from build123d import *

# Parameters (mm, degrees)
EXTRUDE_1_DEPTH     = 5
EXTRUDE_2_DEPTH     = 6
EXTRUDE_3_DEPTH     = 6
SKETCH_4_R          = 8
CUT_EXTRUDE_1_DEPTH = 39.963875359


with BuildPart() as part:
    # 草图1 → 凸台-拉伸1 (new, symmetric)
    with BuildSketch(Plane.XY):
        with BuildLine():
            ThreePointArc((17.364205719, 2.386345678), (19.534538398, -5.841979928), (27.889014085, -7.460133888))
            ThreePointArc((27.889014085, -7.460133888), (32.219400839, -3.446774076), (32.617548437, 2.443963137))
            ThreePointArc((32.617548437, 2.443963137), (24.999999643, 9.4528e-05), (17.364205719, 2.386345678))
        make_face()
        with BuildLine():
            ThreePointArc((-0.737142857, 14.981876398), (-10.864095518, 10.342699288), (-15, 0))
            Line((-15, 0), (-15, -13.8873794))
            ThreePointArc((-15, -13.8873794), (-14.015653031, -16.10934764), (-11.708571429, -16.873190745))
            ThreePointArc((-11.708571429, -16.873190745), (8.410971794, -13.51595237), (27.889014085, -7.460133888))
            ThreePointArc((27.889014085, -7.460133888), (19.534538398, -5.841979928), (17.364205719, 2.386345678))
            ThreePointArc((17.364205719, 2.386345678), (13.547023493, 6.501980338), (11.776397664, 11.828725402))
            ThreePointArc((11.776397664, 11.828725402), (10.960769899, 13.5814964), (9.245219778, 14.472755399))
            ThreePointArc((9.245219778, 14.472755399), (4.266792486, 14.97738476), (-0.737142857, 14.981876398))
        make_face()
    extrude(amount=EXTRUDE_1_DEPTH, both=True)

    # 草图2 → 凸台-拉伸2 (add, symmetric)
    with BuildSketch(Plane.XY):
        with BuildLine():
            ThreePointArc((-15, 0), (3.625161022, -14.555349792), (13.247761009, 7.03539823))
            ThreePointArc((13.247761009, 7.03539823), (7.410500688, 13.041644051), (-0.737142857, 14.981876398))
            ThreePointArc((-0.737142857, 14.981876398), (-10.864095518, 10.342699288), (-15, 0))
        make_face()
    extrude(amount=EXTRUDE_2_DEPTH, both=True)

    # 草图3 → 凸台-拉伸3 (add, symmetric)
    with BuildSketch(Plane.XY):
        with BuildLine():
            ThreePointArc((17.364205719, 2.386345678), (25.030218713, -7.999942927), (32.617548437, 2.443963137))
            ThreePointArc((32.617548437, 2.443963137), (24.999999643, 9.4528e-05), (17.364205719, 2.386345678))
        make_face()
    extrude(amount=EXTRUDE_3_DEPTH, both=True)

    # 草图4 → 切除-拉伸1 (cut, through all)
    with BuildSketch(Plane.XY.offset(6)):
        Circle(SKETCH_4_R)
    extrude(amount=-CUT_EXTRUDE_1_DEPTH, mode=Mode.SUBTRACT)


solid = part.part
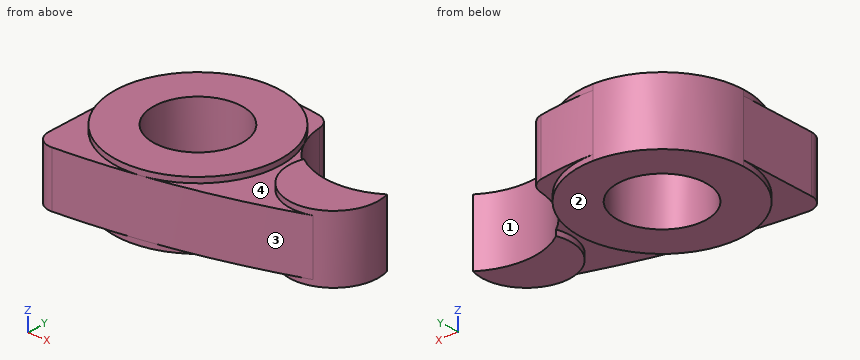
Geometry: final body of the model. Coordinates: model frame, mm. Face numbers are marked on the shaded views. Give positions to 0.01 mm unless a question says otherwise; leave off trailing zeros. Write each loop counter-clockwise with the first axis right and the second up, starting at its lowest first coordinate (ties: lowest second). Pieces come first, ordered by that corner, then holes. Notation, with made-up numbers: (41, 57.5) -> (84, 57.5) arc R14 ccw to (84, 69.5) -> close; hole circle Ø2 at (87, -24). An arc over 180 degrees is marked (long way). Answer as a JSON object with one key per item and string values.
1. Ray query, probe 1 along Z at (x, y) = (15.5, -3.5); probe 2 along Y at (x, z) = (0, -0.25); probe 3 along Y at (x, z) = (-7, 4). Return the intervals inside material, ascending. Write a range as from..to.
Ans:
{"probe 1": "z = -5..5", "probe 2": "y = -15.26..-8, 8..15.01", "probe 3": "y = -16.34..-3.87, 3.87..13.27"}
2. Contact query for flat-ended pins moving along their axis: pin 1 (2 mm diameter, centred on y = 5.5, z = -2.5, fed in from +X); pin 2 (4 mm diameter, centred on x = 16.5, z = 4, fed in from +Y). Output: stop coordinate, or through.
Ans:
{"pin 1": "stops at x = 15", "pin 2": "stops at y = 5.1"}
3. Cut plane A-A on z = -0.5. Output: boundary loops of the cut face in (x, y), and give its area (3 significant figures).
Ans:
{"outline": "(-15, -13.89) arc R3 ccw to (-11.71, -16.87) arc R150 ccw to (27.89, -7.46) arc R8 ccw to (32.62, 2.44) arc R13.25 cw to (11.78, 11.83) arc R3 ccw to (9.25, 14.47) arc R50 ccw to (-0.74, 14.98) arc R15 ccw to (-15, 0) -> close; hole circle Ø16 at (0, 0)", "area": "792 mm^2"}
4. Mould query, pull axis X, two halves, no side actions, for the marked faces 1, 2, 3 and 4. Classes: pulls with the +X half, pulls with the -X half, needs draft (parallel to the pull), parting line crosses it, or undercut.
Ans:
{"face 1": "undercut", "face 2": "needs draft", "face 3": "pulls with the +X half", "face 4": "undercut"}
5. Cut plane B-B on x = 5. Output: boundary loops of the cut face in (y, z) (3 decimals).
Ans:
{"outline": "(-14.285, -5) -> (-14.142, -5) -> (-14.142, -6) -> (-6.245, -6) -> (-6.245, 6) -> (-14.142, 6) -> (-14.142, 5) -> (-14.285, 5) -> close; (6.245, -6) -> (14.142, -6) -> (14.142, -5) -> (14.935, -5) -> (14.935, 5) -> (14.142, 5) -> (14.142, 6) -> (6.245, 6) -> close"}
6. Cut plane D-D on x = 22.5. Output: boundary loops of the cut face in (y, z).
Ans:
{"outline": "(-9.43, -5) -> (-7.6, -5) -> (-7.6, -6) -> (0.23, -6) -> (0.23, 6) -> (-7.6, 6) -> (-7.6, 5) -> (-9.43, 5) -> close"}
